```python
from build123d import *

# Parameters (mm, degrees)
SKETCH1_W           = 240
SKETCH1_H           = 85
BOSS_EXTRUDE1_DEPTH = 25
SKETCH2_W           = 236
SKETCH2_H           = 81
CUT_EXTRUDE1_DEPTH  = 23
SKETCH3_W           = 240
SKETCH3_H           = 85
SKETCH3_W_2         = 238
SKETCH3_H_2         = 83
CUT_EXTRUDE2_DEPTH  = 2
SKETCH5_R           = 4
SKETCH5_W           = 20
SKETCH5_H           = 10
BOSS_EXTRUDE2_DEPTH = 7
SKETCH6_R           = 1.5
CUT_EXTRUDE3_DEPTH  = 5
SKETCH7_R           = 3.5
BOSS_EXTRUDE3_DEPTH = 15
SKETCH8_R           = 1.25
CUT_EXTRUDE4_DEPTH  = 7
FILLET1_R           = 0.2
FILLET2_R           = 1


with BuildPart() as part:
    # Sketch1 → Boss-Extrude1 (new body)
    with BuildSketch(Plane(origin=(0, 0, 0), x_dir=(1, 0, 0), z_dir=(0, 1, 0))):
        Rectangle(SKETCH1_W, SKETCH1_H)
    extrude(amount=BOSS_EXTRUDE1_DEPTH)

    # Sketch2 → Cut-Extrude1 (cut)
    with BuildSketch(Plane(origin=(0, 25, 0), x_dir=(1, 0, 0), z_dir=(0, 1, 0))):
        Rectangle(SKETCH2_W, SKETCH2_H)
    extrude(amount=-CUT_EXTRUDE1_DEPTH, mode=Mode.SUBTRACT)

    # Sketch3 → Cut-Extrude2 (cut)
    with BuildSketch(Plane(origin=(0, 25, 0), x_dir=(1, 0, 0), z_dir=(0, 1, 0))):
        Rectangle(SKETCH3_W, SKETCH3_H)
        Rectangle(SKETCH3_W_2, SKETCH3_H_2, mode=Mode.SUBTRACT)
    extrude(amount=-CUT_EXTRUDE2_DEPTH, mode=Mode.SUBTRACT)

    # Sketch5 → Boss-Extrude2 (add)
    with BuildSketch(Plane(origin=(0, 2, 0), x_dir=(1, 0, 0), z_dir=(0, 1, 0))):
        with Locations(Location((-99.5, 20.5, 0), (0, 0, 270))):
            Circle(SKETCH5_R)
        with Locations(Location((103, 20.5, 0), (0, 0, 270))):
            Circle(SKETCH5_R)
        with Locations((-33, 20.5)):
            Rectangle(SKETCH5_W, SKETCH5_H)
        with Locations((27, 20.5)):
            Rectangle(SKETCH5_W, SKETCH5_H)
    extrude(amount=BOSS_EXTRUDE2_DEPTH)

    # Sketch6 → Cut-Extrude3 (cut)
    with BuildSketch(Plane(origin=(0, 9, 0), x_dir=(1, 0, 0), z_dir=(0, 1, 0))):
        with Locations(Location((-99.5, 20.5, 0), (0, 0, 270))):
            Circle(SKETCH6_R)
        with Locations(Location((103, 20.5, 0), (0, 0, 270))):
            Circle(SKETCH6_R)
    extrude(amount=-CUT_EXTRUDE3_DEPTH, mode=Mode.SUBTRACT)

    # Sketch7 → Boss-Extrude3 (add)
    with BuildSketch(Plane(origin=(0, 2, 0), x_dir=(1, 0, 0), z_dir=(0, 1, 0))):
        with Locations(Location((72, 1.5, 0), (0, 0, 270))):
            Circle(SKETCH7_R)
        with Locations(Location((-69.5, -29.5, 0), (0, 0, 270))):
            Circle(SKETCH7_R)
        with Locations(Location((-69.5, 1.5, 0), (0, 0, 270))):
            Circle(SKETCH7_R)
    extrude(amount=BOSS_EXTRUDE3_DEPTH)

    # Sketch8 → Cut-Extrude4 (cut)
    with BuildSketch(Plane(origin=(0, 17, 0), x_dir=(1, 0, 0), z_dir=(0, 1, 0))):
        with Locations(Location((72, 1.5, 0), (0, 0, 270))):
            Circle(SKETCH8_R)
        with Locations(Location((-69.5, -29.5, 0), (0, 0, 270))):
            Circle(SKETCH8_R)
        with Locations(Location((-69.5, 1.5, 0), (0, 0, 270))):
            Circle(SKETCH8_R)
    extrude(amount=-CUT_EXTRUDE4_DEPTH, mode=Mode.SUBTRACT)

    # Fillet1
    fillet1_edges = [part.edges().sort_by_distance(p)[0] for p in [
        (-23, 5.5, -15.5),
        (-23, 5.5, -25.5),
        (-43, 5.5, -25.5),
        (-43, 5.5, -15.5),
        (-23, 9, -20.5),
        (-33, 9, -25.5),
        (-43, 9, -20.5),
        (-33, 9, -15.5),
        (37, 5.5, -15.5),
        (37, 5.5, -25.5),
        (17, 5.5, -25.5),
        (17, 5.5, -15.5),
        (37, 9, -20.5),
        (27, 9, -25.5),
        (17, 9, -20.5),
        (27, 9, -15.5),
    ]]
    fillet(fillet1_edges, radius=FILLET1_R)

    # Fillet2
    fillet2_edges = [part.edges().sort_by_distance(p)[0] for p in [
        (120, 11.5, 42.5),
        (-120, 11.5, 42.5),
        (-120, 11.5, -42.5),
        (120, 11.5, -42.5),
    ]]
    fillet(fillet2_edges, radius=FILLET2_R)


solid = part.part
```
Model file for the job. Use its own axes, mm. A direction names the side the tool comes from. Give positions to 0.01 mm unless a question says otherwise; leave off trailing zeros. Order: outer loops, then holes, each group sorted by start corner. A loop starts at its lowest first (then second) coordinate and runs counter-clockwise, first axis right, second up.
1) Saw through at D-D, the plane x = 8. Write the cut outline in (y, z).
2) Pin check, flat tips, straight feed: pin 1 (3.5 mm diameter, centred on x = 103.5, z = -20.5, fed in from +Y); pin 2 (0.8 mm diameter, centred on x = 72, z = -1.5, fed in from +Y); pin 3 (3 mm diameter, centred on x = -79.5, z = 18, fed in from +Y). Stop position of each tip, or through.
3) 3-axis set-ups, long thin cutter, end or side, ignore diameter. For faces 1 (the flat face through (27, 5, -15.5)), 2 (the flat face through (-2, 0, -1)): which of +Z, -Z, +X, -X, +Y, -Y reach the whole face in a straight line?
4) Mould opens along X. For faces 3 (the flat face through (-2, 11, 42.5)), 4 (the flat face through (37, 5, -20)) say: +X half, -X half, draft (parallel to the pull), parting line (faces both ways), or undercut.
5) Saw through at C-C, the plane z = 9.5. Write the cut outline in (x, y), then the cut area to 3 significant figures.
6) Saw through at A-A, the plane y = 20.75. Write the cut outline in (x, z).
7) Wall check: probe 1 along X at (y, z) = (13.5, -1.5); probe 2 along X at (y, z) = (12.5, -33.5); probe 3 along Z at (x, y) = (0.5, 9.75). Give the ranges that are in metal, low to high.
8) Saw through at B-B, the plane x = -36.5. Write the cut outline in (y, z), then the cut area to 3 significant figures.
Computed:
1. outline: (0, -42.5) - (23, -42.5) - (23, -41.5) - (25, -41.5) - (25, -40.5) - (2, -40.5) - (2, 40.5) - (25, 40.5) - (25, 41.5) - (23, 41.5) - (23, 42.5) - (0, 42.5) - close
2. pin 1: stops at y = 9
2. pin 2: stops at y = 10
2. pin 3: stops at y = 2
3. face 1: +Y
3. face 2: +Z, -Z, +X, -X, -Y
4. face 3: draft
4. face 4: undercut
5. outline: (-120, 0) - (120, 0) - (120, 23) - (119, 23) - (119, 25) - (118, 25) - (118, 2) - (-118, 2) - (-118, 25) - (-119, 25) - (-119, 23) - (-120, 23) - close
5. area: 568 mm2
6. outline: (-120, -41.5) arc R1 ccw to (-119, -42.5) - (119, -42.5) arc R1 ccw to (120, -41.5) - (120, 41.5) arc R1 ccw to (119, 42.5) - (-119, 42.5) arc R1 ccw to (-120, 41.5) - close; hole (-118, -40.5) - (118, -40.5) - (118, 40.5) - (-118, 40.5) - close
7. probe 1: x = -120 to -118, -73 to -70.75, -68.25 to -66, 68.5 to 70.75, 73.25 to 75.5, 118 to 120
7. probe 2: x = -120 to -118, 118 to 120
7. probe 3: z = -42.5 to -40.5, 40.5 to 42.5
8. outline: (0, -42.5) - (23, -42.5) - (23, -41.5) - (25, -41.5) - (25, -40.5) - (2, -40.5) - (2, -25.5) - (8.8, -25.5) arc R0.2 ccw to (9, -25.3) - (9, -15.7) arc R0.2 ccw to (8.8, -15.5) - (2, -15.5) - (2, 40.5) - (25, 40.5) - (25, 41.5) - (23, 41.5) - (23, 42.5) - (0, 42.5) - close
8. area: 328 mm2
